Check sheet for the drawn part. Datum: minimum x, y, z corner. Units: mm. Give positions to 0.01 mm unless a question says otherwise; leave off trailing zeros. Order: outer loops, then holes, each group sorted by start corner. A loop starts at its lowest first (then second) coordinate and runs counter-clockwise, first axis right, second up.
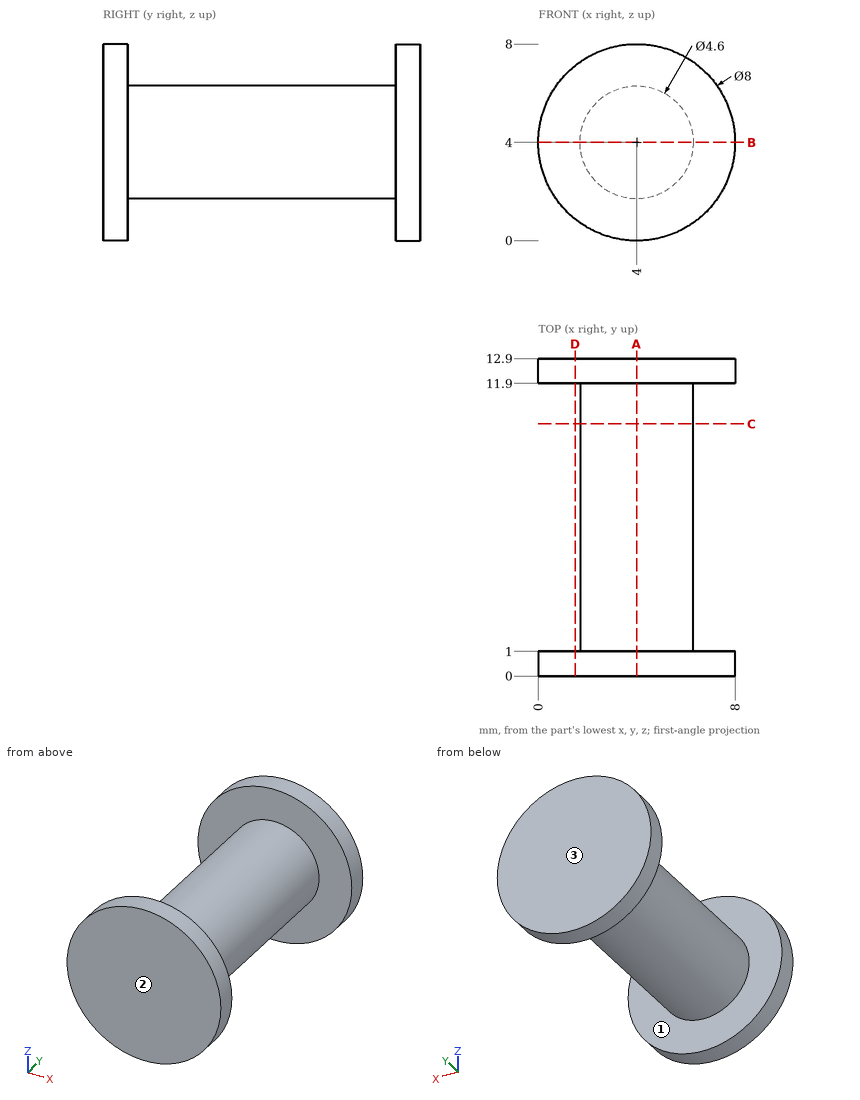
(1) Release check for a two-part mould opening along Y. For the marked faces 1, 2 and 3 record: pulls with the +Y half, pulls with the -Y half, needs draft (parallel to the pull), parting line crosses it, or undercut.
Solved:
face 1: undercut
face 2: pulls with the -Y half
face 3: pulls with the +Y half
(2) Scan lines: line 1 (Y direction, x = 5.75, z = 6.5); line 2 (X direction, y = 5.25, z = 4). Record each from-to range of solid material in increasing order.
Solved:
line 1: y = 0 to 1, 11.9 to 12.9
line 2: x = 1.7 to 6.3
(3) Section check B-B, the plane z = 4. Enter the section's corners in (x, y), then the cut area to 3 significant figures.
Solved:
outline: (0, 0) - (8, 0) - (8, 1) - (6.3, 1) - (6.3, 11.9) - (8, 11.9) - (8, 12.9) - (0, 12.9) - (0, 11.9) - (1.7, 11.9) - (1.7, 1) - (0, 1) - close
area: 66.1 mm2
(4) Go/stop test with flat-tipped pins: pin 1 (1.5 mm diameter, centred on x = 2, y = 7, fed in from -Z); pin 2 (4 mm diameter, centred on y = 9, z = 6, fed in from -X); pin 3 (1.5 mm diameter, centred on y = 9.5, z = 4.5, fed in from +X). Record where each tip stops, or that it passes through.
Solved:
pin 1: stops at z = 2.07
pin 2: stops at x = 1.7
pin 3: stops at x = 6.3
(5) Section check C-C, the plane y = 10.25. Enter the section's corners in (x, z).
Solved:
outline: circle Ø4.6 at (4, 4)
(6) Section check D-D, the plane x = 1.5. Enter the section's corners in (y, z).
Solved:
outline: (0, 0.88) - (1, 0.88) - (1, 7.12) - (0, 7.12) - close; (11.9, 0.88) - (12.9, 0.88) - (12.9, 7.12) - (11.9, 7.12) - close
(7) Section check A-A, the plane x = 4. Enter the section's corners in (y, z).
Solved:
outline: (0, 0) - (1, 0) - (1, 1.7) - (11.9, 1.7) - (11.9, 0) - (12.9, 0) - (12.9, 8) - (11.9, 8) - (11.9, 6.3) - (1, 6.3) - (1, 8) - (0, 8) - close
